Build history of the part. All positions in model axes, mm. A direction names the side the tool comes from. Round coordinates to 2 decimals unless told otherwise and drop trailing zeros. Order: outer loops, then holes, each group sorted by start corner. A loop starts at its lowest first (then second) coordinate and runs counter-clockwise, first axis right, second up. Notation, with made-up numbers: (44, 84.25) - (90, 84.25) arc R24 cw to (90, 105.25) - close; hole circle Ø4 at (-7.75, 73). An arc over 180 degrees is marked (long way). Write each question's results on one line, items separated by ' | '. Start each with the question number.
```python
from build123d import *

# Parameters (mm, degrees)
SKETCH1_W      = 12
SKETCH1_H      = 11
EXTRUDE1_DEPTH = 5
SKETCH2_W      = 12
SKETCH2_H      = 5
EXTRUDE2_DEPTH = 82.76
SKETCH3_W      = 12
SKETCH3_H      = 11
EXTRUDE3_DEPTH = 5
EXTRUDE4_REACH = 95.116
SKETCH5_R      = 1.5
SKETCH8_W      = 6
SKETCH8_H      = 8
EXTRUDE5_DEPTH = 5
SKETCH9_R      = 1.5
EXTRUDE6_DEPTH = 5
FILLET1_R      = 5


with BuildPart() as part:
    # Sketch1 → Extrude1 (new body)
    with BuildSketch(Plane.XY):
        Rectangle(SKETCH1_W, SKETCH1_H)
    extrude(amount=EXTRUDE1_DEPTH)

    # Sketch2 → Extrude2 (add)
    with BuildSketch(Plane.XY.offset(5)):
        with Locations((0, 3)):
            Rectangle(SKETCH2_W, SKETCH2_H)
    extrude(amount=EXTRUDE2_DEPTH)

    # Sketch3 → Extrude3 (add)
    with BuildSketch(Plane.XY.offset(87.76)):
        Rectangle(SKETCH3_W, SKETCH3_H)
    extrude(amount=EXTRUDE3_DEPTH)

    # Extrude4: up to this face of the body (flat: up to its plane)
    extrude4_end = Plane(part.part.faces().sort_by_distance((0, 0, 92.76))[0])
    # Sketch5 → Extrude4 (cut, up to the picked face)
    with BuildSketch(Plane(origin=(0, 0, 0), x_dir=(-1, 0, 0), z_dir=(0, 0, -1)), mode=Mode.PRIVATE) as extrude4_sk1:
        with Locations(Location((-3, -2.5, 0), (0, 0, 180))):
            Circle(SKETCH5_R)
    extrude4_tool1 = split(extrude(extrude4_sk1.sketch, amount=-EXTRUDE4_REACH, mode=Mode.PRIVATE), bisect_by=extrude4_end, keep=Keep.BOTH, mode=Mode.PRIVATE)
    # Sketch5 → Extrude4 (cut, up to the picked face)
    with BuildSketch(Plane(origin=(0, 0, 0), x_dir=(-1, 0, 0), z_dir=(0, 0, -1)), mode=Mode.PRIVATE) as extrude4_sk2:
        with Locations(Location((3, -2.5, 0), (0, 0, 180))):
            Circle(SKETCH5_R)
    extrude4_tool2 = split(extrude(extrude4_sk2.sketch, amount=-EXTRUDE4_REACH, mode=Mode.PRIVATE), bisect_by=extrude4_end, keep=Keep.BOTH, mode=Mode.PRIVATE)
    add(extrude4_tool1.solids().sort_by(Axis((3, -2.5, 0), (0, 0, 1)))[0], mode=Mode.SUBTRACT)
    add(extrude4_tool2.solids().sort_by(Axis((-3, -2.5, 0), (0, 0, 1)))[0], mode=Mode.SUBTRACT)

    # Sketch8 → Extrude5 (cut)
    with BuildSketch(Plane(origin=(0, 5.5, 0), x_dir=(1, 0, 0), z_dir=(0, 1, 0))):
        with Locations((-3, -14)):
            Rectangle(SKETCH8_W, SKETCH8_H)
    extrude(amount=-EXTRUDE5_DEPTH, mode=Mode.SUBTRACT)

    # Sketch9 → Extrude6 (cut)
    with BuildSketch(Plane(origin=(0, 5.5, 0), x_dir=(1, 0, 0), z_dir=(0, 1, 0))):
        with Locations(Location((-3, -22, 0), (0, 0, 270))):
            Circle(SKETCH9_R)
        with Locations(Location((3, -22, 0), (0, 0, 270))):
            Circle(SKETCH9_R)
        with Locations(Location((3, -74.26, 0), (0, 0, 270))):
            Circle(SKETCH9_R)
        with Locations(Location((-3, -74.26, 0), (0, 0, 270))):
            Circle(SKETCH9_R)
    extrude(amount=-EXTRUDE6_DEPTH, mode=Mode.SUBTRACT)

    # Fillet1
    fillet1_edges = [part.edges().sort_by_distance(p)[0] for p in [
        (0, 5.5, 92.76),
        (0, 5.5, 0),
    ]]
    fillet(fillet1_edges, radius=FILLET1_R)


solid = part.part
```
1. Mould opens along X. For faces 1 (the face through (-2.31, -1.17, 2.46)), 2 (the face through (0.08, 4.07, 1.5)), 3 (the face through (3.69, -1.17, 90.22)), 4 (the face through (6, 2, 46)) say: pulls with the +X half, pulls with the -X half, needs draft (parallel to the pull), parting line crosses it, or undercut.
2. Cut at B-B (y = -2.5). List the corners of the cut face in (x, z).
3. Flat gauge pins, fed straight in: pin 1 Ø1.5 at (x, y) = (-3, 2) entering from -Z; pin 2 Ø2 at (x, z) = (4, 17) entering from -Y; pin 3 Ø2.5 at (y, z) = (3, 13.5) entering from -X; pin 4 Ø2.5 at (x, z) = (3, 74.26) entering from +Y. Where does each tip first touch, or does it go through?
4. 3-axis set-ups, long thin cutter, end or side, ignore diameter. For faces 5 (the face through (0, 0.5, 46)), 6 (the face through (0, 3, 14)), 7 (the face through (0, 5.5, 46)): which of +Z, -Z, +X, -X, +Y, -Y reach the whole face in a straight line?
5. Cut at C-C (x = 3). List the corners of the cut face in (y, z), plus the area to 3 significant figures.
6. Cut at D-D (y = 2.5). List the corners of the cut face in (x, z), plus the area to 3 significant figures.
7. Cut at A-A (z = 22). List the corners of the cut face in (x, y), plus the area to 3 significant figures.
8. Wall check: line 1 (X direction, y = -2.5, z = 89.5); line 2 (Z direction, x = 2.5, y = -4.5); line 3 (Z direction, x = -5.5, y = 0.75). Give the ranges that are in metal, low to high. Write a range as from..to.
A:
1) face 1: undercut | face 2: needs draft | face 3: undercut | face 4: pulls with the +X half
2) outline: (-6, 0) - (-4.5, 0) - (-4.5, 5) - (-6, 5) - close; (-6, 87.76) - (-4.5, 87.76) - (-4.5, 92.76) - (-6, 92.76) - close; (-1.5, 0) - (1.5, 0) - (1.5, 5) - (-1.5, 5) - close; (-1.5, 87.76) - (1.5, 87.76) - (1.5, 92.76) - (-1.5, 92.76) - close; (4.5, 0) - (6, 0) - (6, 5) - (4.5, 5) - close; (4.5, 87.76) - (6, 87.76) - (6, 92.76) - (4.5, 92.76) - close
3) pin 1: stops at z = 0.06 | pin 2: stops at y = 0.5 | pin 3: stops at x = 0 | pin 4: passes through
4) face 5: +X, -X, -Y | face 6: -X, +Y, -Y | face 7: +Z, -Z, +X, -X, +Y
5) outline: (-5.5, 0) - (-4, 0) - (-4, 5) - (-5.5, 5) - close; (-5.5, 87.76) - (-4, 87.76) - (-4, 92.76) - (-5.5, 92.76) - close; (-1, 0) - (0.5, 0) arc R5 ccw to (5.5, 5) - (5.5, 20.5) - (0.5, 20.5) - (0.5, 5) - (-1, 5) - close; (-1, 87.76) - (0.5, 87.76) - (0.5, 75.76) - (5.5, 75.76) - (5.5, 87.76) arc R5 ccw to (0.5, 92.76) - (-1, 92.76) - close; (0.5, 23.5) - (5.5, 23.5) - (5.5, 72.76) - (0.5, 72.76) - close | area: 453 mm^2
6) outline: (-6, 0.42) - (6, 0.42) - (6, 92.34) - (-6, 92.34) - (-6, 18) - (0, 18) - (0, 10) - (-6, 10) - close; hole circle Ø3 at (-3, 22); hole circle Ø3 at (-3, 74.26); hole circle Ø3 at (3, 22); hole circle Ø3 at (3, 74.26) | area: 1,030 mm^2
7) outline: (-6, 0.5) - (-4.5, 0.5) - (-4.5, 5.5) - (-6, 5.5) - close; (-1.5, 0.5) - (1.5, 0.5) - (1.5, 5.5) - (-1.5, 5.5) - close; (4.5, 0.5) - (6, 0.5) - (6, 5.5) - (4.5, 5.5) - close | area: 30.0 mm^2
8) line 1: x = -6..-4.5, -1.5..1.5, 4.5..6 | line 2: z = 0..5, 87.76..92.76 | line 3: z = 0.01..10, 18..92.75
